Can you work these out from the model? Positions are in its coordinate system, mm. A direction names the side the tool comes from. Round coordinates to 2 decimals unless told otherwise and drop trailing zeros. Loops run counter-clockwise (first coordinate to the right, second up) from the corner with the lowest first, then second, coordinate; pieces in that order, holes last. Notation, with made-up numbers: (56, 10.25) -> (76, 10.25) arc R20 cw to (76, 33.25) -> close; hole circle Ø5 at (-19, 27). An arc over 180 degrees is marked (long way). Write item = value, one per line.
from build123d import *

# Parameters (mm, degrees)
F1_DEPTH = 1.5
F3_DEPTH = 13.8
F4_W     = 14.5
F4_H     = 12.8
F5_DEPTH = 2
F6_W     = 2
F6_H     = 2
F7_DEPTH = 6
F8_R     = 4


with BuildPart() as f1:
    # F0 (on Top) → F1 (new body)
    with BuildSketch(Plane.XY):
        Polygon((2.435753, 14.841201), (-20.564247, 14.841201), (-20.564247, -2.158799), (-18.564247, -2.158799), (-18.564247, -4.158799), (-16.564247, -12.658799), (-16.564247, -23.158799), (2.435753, -23.158799), align=None)
    extrude(amount=F1_DEPTH)

    # F2 (on face) → F3 (join)
    with BuildSketch(Plane(origin=(0, 0, 0), x_dir=(1, 0, 0), z_dir=(0, 0, -1))):
        Polygon((-14.864247, 23.158799), (-16.564247, 23.158799), (-16.564247, 12.658799), (-18.564247, 4.158799), (-18.564247, 2.158799), (-20.564247, 2.158799), (-20.564247, -14.841201), (-16.964247, -14.841201), (-16.964247, 3.536493), (-14.864247, 12.461493), align=None)
    extrude(amount=F3_DEPTH)

    # F4 (on face) → F5 (join)
    with BuildSketch(Plane(origin=(-20.564247, 0, 0), x_dir=(0, -1, 0), z_dir=(-1, 0, 0))):
        with Locations((-7.591201, -4.9)):
            Rectangle(F4_W, F4_H)
    extrude(amount=F5_DEPTH)

    # F6 (on face) → F7 (join)
    with BuildSketch(Plane(origin=(0, 14.841201, 0), x_dir=(-1, 0, 0), z_dir=(0, 1, 0))):
        with Locations((19.764247, -6.15)):
            Rectangle(F6_W, F6_H)
    extrude(amount=F7_DEPTH)

    # F8
    f8_edges = [f1.edges().sort_by_distance(p)[0] for p in [
        (-15.714247, -23.158799, -13.8),
    ]]
    fillet(f8_edges, radius=F8_R)


solid = f1.part
1. Suppose I cut it at A-A, the plane y = 6.5. List the corners of the cut face in (x, z) for me.
Entries:
outline = (-22.56, -11.3) -> (-20.56, -11.3) -> (-20.56, -13.8) -> (-16.96, -13.8) -> (-16.96, 0) -> (2.44, 0) -> (2.44, 1.5) -> (-22.56, 1.5) -> close
2. For faces 1 (the flat face through (-20, 18, -5.15)), 2 (the flat face through (-22, 8, -11.3)), 3 (the flat face through (-20, 18, -7.15)), 4 (the flat face through (-20.764, 18, -6)), 5 (the flat face through (-18.564, -3, -6)), which set-ups out of +Z, -Z, +X, -X, +Y, -Y let a thin tool reach every point of the face, with its end or its side?
Entries:
face_1 = +Z, +X, -X, +Y
face_2 = -Z, -X, +Y, -Y
face_3 = -Z, +X, -X, +Y
face_4 = +Z, -Z, -X, +Y
face_5 = +Z, -Z, -X, -Y
3. I'm going to push flat-ended pins straight in: pin 1 (0.6 mm diameter, centred on x = -19, z = -2.5, fed in from -Y); pin 2 (7.5 mm diameter, centred on x = -6.5, z = -4.5, fed in from +Y); pin 3 (1.6 mm diameter, centred on y = -3, z = -8, fed in from -X); pin 4 (1 mm diameter, centred on y = 17.5, z = -6, fed in from -X). Where does each tip first touch, or does it pass through?
Entries:
pin_1 = -2.16
pin_2 = through
pin_3 = -18.56
pin_4 = -20.76
4. I need wall thicknesses on line 1 (X direction, y = 15, z = -6.75); line 2 (X direction, y = -15.5, z = -6); line 3 (Z direction, x = -6.75, y = 4). Which ranges of each line are inside material? Lowest first, please. Write a range as [from, to].
Entries:
line_1 = [-20.76, -18.76]
line_2 = [-16.56, -14.86]
line_3 = [0, 1.5]
5. Suppose I cut it at B-B, the plane z = -2. List the corners of the cut face in (x, y) for me, and give its area (3 significant figures).
Entries:
outline = (-22.56, 0.34) -> (-20.56, 0.34) -> (-20.56, -2.16) -> (-18.56, -2.16) -> (-18.56, -4.16) -> (-16.56, -12.66) -> (-16.56, -23.16) -> (-14.86, -23.16) -> (-14.86, -12.46) -> (-16.96, -3.54) -> (-16.96, 14.84) -> (-22.56, 14.84) -> close
area = 126 mm²
6. Suppose I cut it at D-D, the plane y = 18. List the corners of the cut face in (x, z) for me.
Entries:
outline = (-20.76, -7.15) -> (-18.76, -7.15) -> (-18.76, -5.15) -> (-20.76, -5.15) -> close
7. Suppose I cut it at C-C, the plane x = -11.75. List the corners of the cut face in (y, z) for me, and give its area (3 significant figures).
Entries:
outline = (-23.16, 0) -> (14.84, 0) -> (14.84, 1.5) -> (-23.16, 1.5) -> close
area = 57.0 mm²
